Design review of the part built by this model. Coordinates are the model's own, in mm. Face numbers are marked on the shaded views. A direction names the side the tool comes from. Round coordinates to 2 decimals unless told otherwise and drop trailing zeros. Order: outer loops, then holes, each group sorted by start corner. A loop starts at its lowest first (then second) coordinate and runs counter-clockwise, first axis right, second up. Notation, with made-up numbers: (43.25, 50.5) - (65.25, 50.5) arc R22 cw to (65.25, 83.5) - close; hole circle Ø6 at (-4, -16.75). An arc over 180 degrees is marked (long way). Use CSV: the item, a comma, the result in double quotes. Start each with the question number.
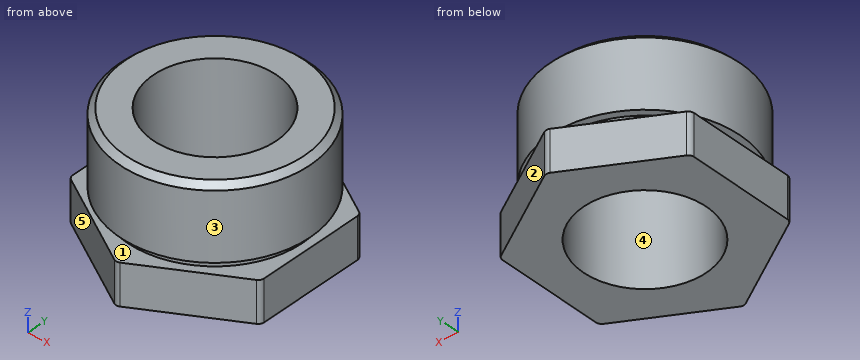
from build123d import *

# Parameters (mm, degrees)
SKETCH1_R           = 32.5
BOSS_EXTRUDE1_DEPTH = 42
CUT_EXTRUDE1_START  = -28
SKETCH2_R           = 32.5
SKETCH2_R_2         = 30
CUT_EXTRUDE1_DEPTH  = 3
BOSS_EXTRUDE2_DEPTH = 14
FILLET1_R           = 2
CHAMFER1_SIZE       = 2
SKETCH4_R           = 21
CUT_EXTRUDE3_DEPTH  = 66.153392256


with BuildPart() as part:
    # Sketch1 → Boss-Extrude1 (new body)
    with BuildSketch(Plane.XY):
        with Locations(Location((0, 0, 0), (0, 0, 180))):
            Circle(SKETCH1_R)
    extrude(amount=BOSS_EXTRUDE1_DEPTH)

    # Sketch2 → Cut-Extrude1 (cut)
    with BuildSketch(Plane.XY.offset(42).offset(CUT_EXTRUDE1_START)):
        with Locations(Location((0, 0, 0), (0, 0, 180))):
            Circle(SKETCH2_R)
        Circle(SKETCH2_R_2, mode=Mode.SUBTRACT)
    extrude(amount=CUT_EXTRUDE1_DEPTH, mode=Mode.SUBTRACT)

    # Sketch3 → Boss-Extrude2 (add)
    with BuildSketch(Plane(origin=(0, 0, 0), x_dir=(-1, 0, 0), z_dir=(0, 0, -1))):
        Polygon((0, -37.828766952), (32.760673174, -18.914383476), (32.760673174, 18.914383476), (0, 37.828766952), (-32.760673174, 18.914383476), (-32.760673174, -18.914383476), align=None)
    extrude(amount=-BOSS_EXTRUDE2_DEPTH)

    # Fillet1
    fillet1_edges = [part.edges().sort_by_distance(p)[0] for p in [
        (0, -37.828766952, 7),
        (32.760673174, -18.914383476, 7),
        (32.760673174, 18.914383476, 7),
        (0, 37.828766952, 7),
        (-32.760673174, 18.914383476, 7),
        (-32.760673174, -18.914383476, 7),
    ]]
    fillet(fillet1_edges, radius=FILLET1_R)

    # Chamfer1
    chamfer1_edges = [part.edges().sort_by_distance(p)[0] for p in [
        (32.5, 0, 42),
    ]]
    chamfer(chamfer1_edges, length=CHAMFER1_SIZE)

    # Sketch4 → Cut-Extrude3 (cut, through all)
    with BuildSketch(Plane.XY.offset(42)):
        Circle(SKETCH4_R)
    extrude(amount=-CUT_EXTRUDE3_DEPTH, mode=Mode.SUBTRACT)


solid = part.part
Q1. Tool access review of the marked faces 1 and 2: name each direction out of +Z, -Z, +X, -X, +Y, -Y from which nothing blocks a thin tool from reaching the whole face with its end or side.
Q2. Clearance check with flat-ended pins moving along their axes: pin 1 (6 mm diameter, centred on x = 2.5, y = -24.5, fed in from -Z); pin 2 (12 mm diameter, centred on x = 21, z = 15, fed in from -Y); pin 3 (8 mm diameter, centred on y = -4, z = 19, fed in from -X); pin 4 (1 mm diameter, centred on x = 10, z = 10.5, fed in from +Y). State where each tip first meets the part, or that it passes through.
Q3. The part is to be moulded in two halves that separate along X. For the marked faces 3, 4 and 5, say which applies: +X half, -X half, draft (parallel to the pull), parting line (faces both ways), or undercut.
Q4. For L1, parallel to Y at x = 0, z = 24; L2, parallel to Z at x = -15, y = 26.5; L3, parallel to Y at x = 0, z = 16.5, list the stretches that pass through material, from the lowest coordinate up. Write a range as [from, to].
Q5. Take a section at C-C (y = 0). State the section outline as (x, z) points, plus the area to 3 significant figures.
Q6. Take a section at B-B (z = 5.5). State the section outline as (x, y) points.
Q7. Take a section at D-D (z = 38). State the section outline as (x, y) points, plus the area to 3 significant figures.
Q8. Take a section at A-A (x = 0). State the section outline as (y, z) points, plus the area to 3 significant figures.
Findings below:
1,face 1,"none"
1,face 2,"+Z, -Z, +X, +Y"
2,pin 1,"stops at z = 0"
2,pin 2,"stops at y = -29.12"
2,pin 3,"stops at x = -32.5"
2,pin 4,"stops at y = 32.34"
3,face 3,"parting line"
3,face 4,"undercut"
3,face 5,"-X half"
4,L1,"y = [-32.5, -21], [21, 32.5]"
4,L2,"z = [0, 14], [17, 42]"
4,L3,"y = [-30, -21], [21, 30]"
5,outline,"(-32.76, 0) - (-21, 0) - (-21, 42) - (-30.5, 42) - (-32.5, 40) - (-32.5, 17) - (-30, 17) - (-30, 14) - (-32.76, 14) - close; (21, 0) - (32.76, 0) - (32.76, 14) - (30, 14) - (30, 17) - (32.5, 17) - (32.5, 40) - (30.5, 42) - (21, 42) - close"
5,area,"954 mm^2"
6,outline,"(-32.76, -17.76) arc R2 ccw to (-31.76, -19.49) - (-1, -37.25) arc R2 ccw to (1, -37.25) - (31.76, -19.49) arc R2 ccw to (32.76, -17.76) - (32.76, 17.76) arc R2 ccw to (31.76, 19.49) - (1, 37.25) arc R2 ccw to (-1, 37.25) - (-31.76, 19.49) arc R2 ccw to (-32.76, 17.76) - close; hole circle Ø42 at (0, 0)"
7,outline,"circle Ø65 at (0, 0); hole circle Ø42 at (0, 0)"
7,area,"1,930 mm^2"
8,outline,"(-37.52, 0) - (-21, 0) - (-21, 42) - (-30.5, 42) - (-32.5, 40) - (-32.5, 17) - (-30, 17) - (-30, 14) - (-37.52, 14) - close; (21, 0) - (37.52, 0) - (37.52, 14) - (30, 14) - (30, 17) - (32.5, 17) - (32.5, 40) - (30.5, 42) - (21, 42) - close"
8,area,"1,090 mm^2"
